Can you work these out from the model? Positions are in its coordinate system, mm. A direction names the side the tool comes from. Give positions to 0.01 mm unless a question says otherwise; leave off trailing zeros. Loops run counter-clockwise (first coordinate to the right, second up) from the corner with the lowest first, then second, coordinate; pieces in that order, holes last. Notation, with made-up numbers: (86.5, -31) -> (130.5, -31) arc R13 ccw to (130.5, -15) -> close; hole circle Ø6 at (67, 69). An arc over 180 degrees is marked (long way). Use CSV: the item, a comma, the result in double quotes.
from build123d import *

# Parameters (mm, degrees)
SKETCH1_R           = 7.5
BOSS_EXTRUDE1_DEPTH = 5
SKETCH2_R           = 1
CUT_EXTRUDE1_DEPTH  = 10
SKETCH3_R           = 2.6
CUT_EXTRUDE2_DEPTH  = 2
BOSS_EXTRUDE3_DEPTH = 5
CIRPATTERN1_DEPTH   = 5


# Read off the part's stored shape, not the designer's step: CirPattern1
with BuildPart() as part:
    # Sketch1 → Boss-Extrude1 (new body)
    with BuildSketch(Plane(origin=(0, 0, 0), x_dir=(1, 0, 0), z_dir=(0, 1, 0))):
        with Locations(Location((0, 0, 0), (0, 0, 270))):
            Circle(SKETCH1_R)
    extrude(amount=BOSS_EXTRUDE1_DEPTH)

    # Sketch2 → Cut-Extrude1 (cut)
    with BuildSketch(Plane(origin=(0, 5, 0), x_dir=(1, 0, 0), z_dir=(0, 1, 0))):
        with Locations(Location((0, 0, 0), (0, 0, 270))):
            Circle(SKETCH2_R)
    extrude(amount=-CUT_EXTRUDE1_DEPTH, mode=Mode.SUBTRACT)

    # Sketch3 → Cut-Extrude2 (cut)
    with BuildSketch(Plane(origin=(0, 5, 0), x_dir=(1, 0, 0), z_dir=(0, 1, 0))):
        with Locations(Location((0, 0, 0), (0, 0, 270))):
            Circle(SKETCH3_R)
    extrude(amount=-CUT_EXTRUDE2_DEPTH, mode=Mode.SUBTRACT)

    # Sketch6 → Boss-Extrude3 (add)
    with BuildSketch(Plane(origin=(0, 0, 0), x_dir=(1, 0, 0), z_dir=(0, 1, 0))):
        with BuildLine():
            ThreePointArc((0.2, 9.9979998), (0, 10), (-0.2, 9.9979998))
            ThreePointArc((-0.2, 9.9979998), (-0.977699989, 8.79848798), (-1.25, 7.395099729))
            ThreePointArc((-1.25, 7.395099729), (0, 7.5), (1.25, 7.395099729))
            ThreePointArc((1.25, 7.395099729), (0.977699989, 8.79848798), (0.2, 9.9979998))
        make_face()
    extrude(amount=BOSS_EXTRUDE3_DEPTH)

    # CirPattern1 outline → CirPattern1 (add)
    with BuildSketch(Plane(origin=(0, 0, 0), x_dir=(1, 0, 0), z_dir=(0, 1, 0))):
        with BuildLine():
            ThreePointArc((-3.607455849, 9.326642606), (-3.927997585, 7.933481138), (-3.703888845, 6.521595466))
            ThreePointArc((-3.703888845, 6.521595466), (-2.565151075, 7.047694656), (-1.354657293, 7.376645825))
            ThreePointArc((-1.354657293, 7.376645825), (-2.090522655, 8.602267319), (-3.2315788, 9.463450663))
            ThreePointArc((-3.2315788, 9.463450663), (-3.420201433, 9.396926208), (-3.607455849, 9.326642606))
        make_face()
        with BuildLine():
            ThreePointArc((-6.579799282, 7.530354667), (-6.404520701, 6.111579386), (-5.711034032, 4.861490542))
            ThreePointArc((-5.711034032, 4.861490542), (-4.820907072, 5.745333324), (-3.795922924, 6.468459566))
            ThreePointArc((-3.795922924, 6.468459566), (-4.906597414, 7.368486264), (-6.273381504, 7.787469711))
            ThreePointArc((-6.273381504, 7.787469711), (-6.427876097, 7.660444431), (-6.579799282, 7.530354667))
        make_face()
        with BuildLine():
            ThreePointArc((-8.758521814, 4.825794819), (-8.1085641, 3.552530962), (-7.029344229, 2.61501811))
            ThreePointArc((-7.029344229, 2.61501811), (-6.495190528, 3.75), (-5.779344229, 4.780081619))
            ThreePointArc((-5.779344229, 4.780081619), (-7.130864111, 5.245957017), (-8.558521814, 5.172204981))
            ThreePointArc((-8.558521814, 5.172204981), (-8.660254038, 5), (-8.758521814, 4.825794819))
        make_face()
        with BuildLine():
            ThreePointArc((-9.880837353, 1.539172895), (-8.834594998, 0.564994875), (-7.499811769, 0.0531359))
            ThreePointArc((-7.499811769, 0.0531359), (-7.386058148, 1.302361332), (-7.065691325, 2.515155283))
            ThreePointArc((-7.065691325, 2.515155283), (-8.495043356, 2.490687933), (-9.811378082, 1.933095996))
            ThreePointArc((-9.811378082, 1.933095996), (-9.84807753, 1.736481777), (-9.880837353, 1.539172895))
        make_face()
        with BuildLine():
            ThreePointArc((-9.811378082, -1.933095996), (-8.495043356, -2.490687933), (-7.065691325, -2.515155283))
            ThreePointArc((-7.065691325, -2.515155283), (-7.386058148, -1.302361332), (-7.499811769, -0.0531359))
            ThreePointArc((-7.499811769, -0.0531359), (-8.834594998, -0.564994875), (-9.880837353, -1.539172895))
            ThreePointArc((-9.880837353, -1.539172895), (-9.84807753, -1.736481777), (-9.811378082, -1.933095996))
        make_face()
        with BuildLine():
            ThreePointArc((-8.558521814, -5.172204981), (-7.130864111, -5.245957017), (-5.779344229, -4.780081619))
            ThreePointArc((-5.779344229, -4.780081619), (-6.495190528, -3.75), (-7.029344229, -2.61501811))
            ThreePointArc((-7.029344229, -2.61501811), (-8.1085641, -3.552530962), (-8.758521814, -4.825794819))
            ThreePointArc((-8.758521814, -4.825794819), (-8.660254038, -5), (-8.558521814, -5.172204981))
        make_face()
        with BuildLine():
            ThreePointArc((-6.273381504, -7.787469711), (-4.906597414, -7.368486264), (-3.795922924, -6.468459566))
            ThreePointArc((-3.795922924, -6.468459566), (-4.820907072, -5.745333324), (-5.711034032, -4.861490542))
            ThreePointArc((-5.711034032, -4.861490542), (-6.404520701, -6.111579386), (-6.579799282, -7.530354667))
            ThreePointArc((-6.579799282, -7.530354667), (-6.427876097, -7.660444431), (-6.273381504, -7.787469711))
        make_face()
        with BuildLine():
            ThreePointArc((-3.2315788, -9.463450663), (-2.090522655, -8.602267319), (-1.354657293, -7.376645824))
            ThreePointArc((-1.354657293, -7.376645824), (-2.565151075, -7.047694656), (-3.703888845, -6.521595466))
            ThreePointArc((-3.703888845, -6.521595466), (-3.927997585, -7.933481138), (-3.607455849, -9.326642606))
            ThreePointArc((-3.607455849, -9.326642606), (-3.420201433, -9.396926208), (-3.2315788, -9.463450663))
        make_face()
        with BuildLine():
            ThreePointArc((0.2, -9.9979998), (0.977699989, -8.79848798), (1.25, -7.395099729))
            ThreePointArc((1.25, -7.395099729), (0, -7.5), (-1.25, -7.395099729))
            ThreePointArc((-1.25, -7.395099729), (-0.977699989, -8.79848798), (-0.2, -9.9979998))
            ThreePointArc((-0.2, -9.9979998), (0, -10), (0.2, -9.9979998))
        make_face()
        with BuildLine():
            ThreePointArc((3.607455849, -9.326642606), (3.927997585, -7.933481138), (3.703888845, -6.521595466))
            ThreePointArc((3.703888845, -6.521595466), (2.565151075, -7.047694656), (1.354657293, -7.376645824))
            ThreePointArc((1.354657293, -7.376645824), (2.090522655, -8.602267319), (3.2315788, -9.463450663))
            ThreePointArc((3.2315788, -9.463450663), (3.420201433, -9.396926208), (3.607455849, -9.326642606))
        make_face()
        with BuildLine():
            ThreePointArc((6.579799282, -7.530354667), (6.404520701, -6.111579386), (5.711034032, -4.861490542))
            ThreePointArc((5.711034032, -4.861490542), (4.820907072, -5.745333324), (3.795922924, -6.468459566))
            ThreePointArc((3.795922924, -6.468459566), (4.906597414, -7.368486264), (6.273381504, -7.787469711))
            ThreePointArc((6.273381504, -7.787469711), (6.427876097, -7.660444431), (6.579799282, -7.530354667))
        make_face()
        with BuildLine():
            ThreePointArc((8.758521814, -4.825794819), (8.1085641, -3.552530962), (7.029344229, -2.61501811))
            ThreePointArc((7.029344229, -2.61501811), (6.495190528, -3.75), (5.779344229, -4.780081619))
            ThreePointArc((5.779344229, -4.780081619), (7.130864111, -5.245957017), (8.558521814, -5.172204981))
            ThreePointArc((8.558521814, -5.172204981), (8.660254038, -5), (8.758521814, -4.825794819))
        make_face()
        with BuildLine():
            ThreePointArc((1.354657293, 7.376645825), (2.565151075, 7.047694656), (3.703888845, 6.521595466))
            ThreePointArc((3.703888845, 6.521595466), (3.927997585, 7.933481138), (3.607455849, 9.326642606))
            ThreePointArc((3.607455849, 9.326642606), (3.420201433, 9.396926208), (3.2315788, 9.463450663))
            ThreePointArc((3.2315788, 9.463450663), (2.090522655, 8.602267319), (1.354657293, 7.376645825))
        make_face()
        with BuildLine():
            ThreePointArc((3.795922924, 6.468459566), (4.820907072, 5.745333324), (5.711034032, 4.861490542))
            ThreePointArc((5.711034032, 4.861490542), (6.404520701, 6.111579386), (6.579799282, 7.530354667))
            ThreePointArc((6.579799282, 7.530354667), (6.427876097, 7.660444431), (6.273381504, 7.787469711))
            ThreePointArc((6.273381504, 7.787469711), (4.906597414, 7.368486264), (3.795922924, 6.468459566))
        make_face()
        with BuildLine():
            ThreePointArc((5.779344229, 4.780081619), (6.495190528, 3.75), (7.029344229, 2.61501811))
            ThreePointArc((7.029344229, 2.61501811), (8.1085641, 3.552530962), (8.758521814, 4.825794819))
            ThreePointArc((8.758521814, 4.825794819), (8.660254038, 5), (8.558521814, 5.172204981))
            ThreePointArc((8.558521814, 5.172204981), (7.130864111, 5.245957017), (5.779344229, 4.780081619))
        make_face()
        with BuildLine():
            ThreePointArc((7.065691325, 2.515155283), (7.386058148, 1.302361332), (7.499811769, 0.0531359))
            ThreePointArc((7.499811769, 0.0531359), (8.834594998, 0.564994875), (9.880837353, 1.539172895))
            ThreePointArc((9.880837353, 1.539172895), (9.84807753, 1.736481777), (9.811378082, 1.933095996))
            ThreePointArc((9.811378082, 1.933095996), (8.495043356, 2.490687933), (7.065691325, 2.515155283))
        make_face()
        with BuildLine():
            ThreePointArc((9.811378082, -1.933095996), (9.84807753, -1.736481777), (9.880837353, -1.539172895))
            ThreePointArc((9.880837353, -1.539172895), (8.834594998, -0.564994875), (7.499811769, -0.0531359))
            ThreePointArc((7.499811769, -0.0531359), (7.386058148, -1.302361332), (7.065691325, -2.515155283))
            ThreePointArc((7.065691325, -2.515155283), (8.495043356, -2.490687933), (9.811378082, -1.933095996))
        make_face()
    extrude(amount=CIRPATTERN1_DEPTH)


solid = part.part
(1) If we section it at C-C, the plane z = -6: Write out the boundary of the cut face in (x, y), then the cut area to 3 significant figures.
Answer sheet:
outline,"(-6.37, 0) -> (6.37, 0) -> (6.37, 5) -> (-6.37, 5) -> close"
area,"63.7 mm2"
(2) If we section it at B-B, the plane x = -2.25: Write out the boundary of the cut face in (y, z).
Answer sheet:
outline,"(0, -8.77) -> (5, -8.77) -> (5, -1.3) -> (3, -1.3) -> (3, 1.3) -> (5, 1.3) -> (5, 8.77) -> (0, 8.77) -> close"
(3) If I drill on L1, parallel to X at y = 2.65, z = 7.5; L2, parallel to X at y = 2.2, z = 0; L3, parallel to X at y = 3.6, z = 6.75, over which ranges is the centre line in solid material (lowest first)? Write a range as from..to.
Answer sheet:
L1,"x = -6.58..-5.18, -3.92..-1.4, -1.25..1.25, 1.4..3.92, 5.18..6.58"
L2,"x = -7.5..-1, 1..7.5"
L3,"x = -6.55..-4.06, -3.78..3.78, 4.06..6.55"
(4) If we section it at D-D, the plane x = 5: Write out the boundary of the cut face in (y, z), then the cut area to 3 significant figures.
Answer sheet:
outline,"(0, -7.42) -> (5, -7.42) -> (5, 7.42) -> (0, 7.42) -> close"
area,"74.2 mm2"
(5) Will these pins go through, and if not, where does the flat tip stop? pin 1 Ø1.2 at (x, z) = (0, 0) entering from -Y (1 decimal); pin 2 Ø1 at (x, y) = (4, 0.5) entering from -Z; pin 3 Ø2 at (x, y) = (5, 3) entering from -Z; pin 4 Ø4 at (x, z) = (-0.5, 0) entering from +Y.
Answer sheet:
pin 1,"passes through"
pin 2,"stops at z = -9.37"
pin 3,"stops at z = -7.75"
pin 4,"stops at y = 3"
(6) If we section it at A-A, the plane z = -0.75: Write out the boundary of the cut face in (x, y), then the cut area to 3 significant figures.
Answer sheet:
outline,"(-9.1, 0) -> (-0.66, 0) -> (-0.66, 3) -> (-2.49, 3) -> (-2.49, 5) -> (-9.1, 5) -> close; (0.66, 0) -> (9.1, 0) -> (9.1, 5) -> (2.49, 5) -> (2.49, 3) -> (0.66, 3) -> close"
area,"77.1 mm2"
(7) We'd pull the mould along Z, two halves only. Please class faces 4 (the face through (-2.08, 2.46, -8.59)), 5 (the face through (-2, 0, 0)), 6 (the face through (8.817, 2.465, -0.554)): released by +Z, released by -Z, zero draft, split by the parting line, or undercut.
Answer sheet:
face 4,"released by -Z"
face 5,"zero draft"
face 6,"undercut"
(8) Which directions (+Z, -Z, +X, -X, +Y, -Y) give clear straight access to the entire face, cutting with the end or side of a thin tool? Please do faces 1 (the face through (0.78, 4.01, 2.48)), 2 (the face through (3.927, 2.465, 7.954)), 3 (the face through (-8.817, 2.465, 0.554)).
Answer sheet:
face 1,"+Y"
face 2,"+Y, -Y"
face 3,"-X, +Y, -Y"
